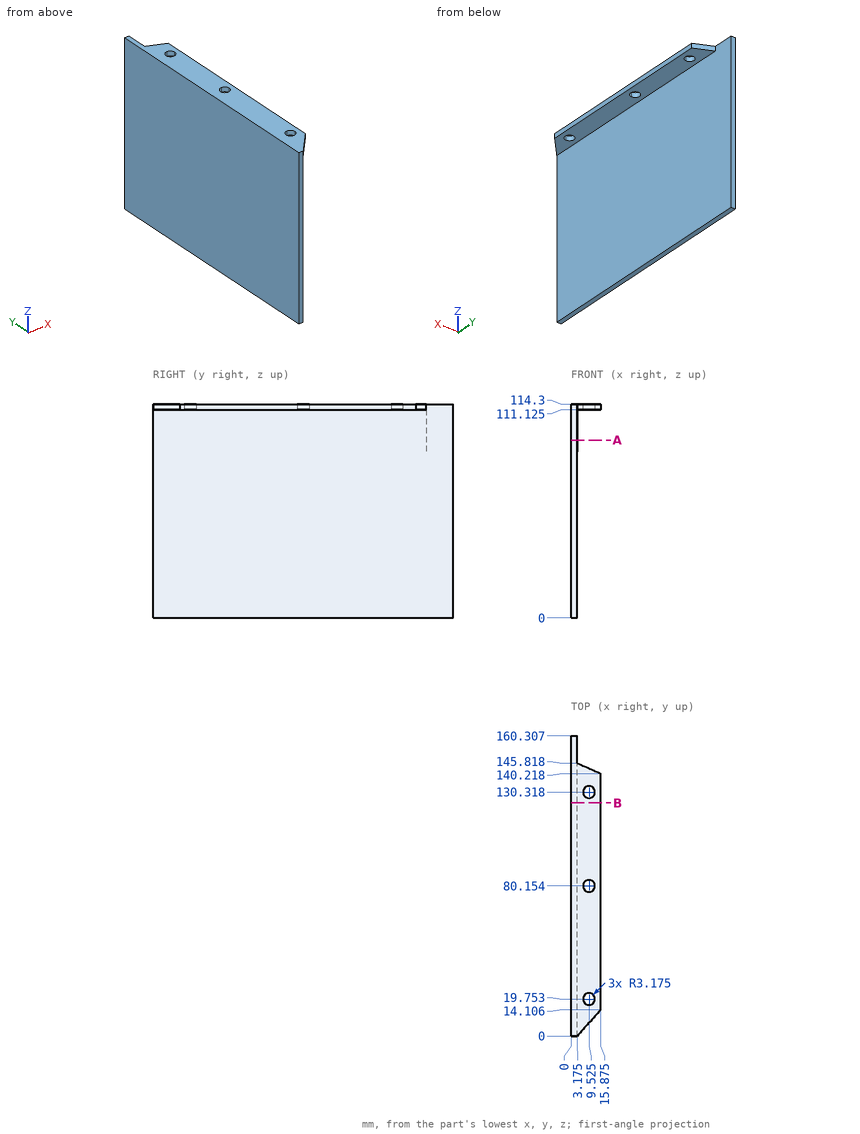
Can you work these out from the drawing? Everything is in mm from the part's minimum corner. Round coordinates to 2 decimals unless told otherwise and drop trailing zeros. Loops run counter-clockwise (first coordinate to the right, second up) from the corner with the lowest first, then second, coordinate; pieces in that order, holes last. Notation, with made-up numbers: (64, 84.25) - (92, 84.25) arc R13 ccw to (92, 99.25) - close; hole circle Ø10 at (22, -19). An arc over 180 degrees is marked (long way). Answer in a Markdown table with one row per item. Add a question column.
(1) I need wall thicknesses on line 1 along Z through (x, y) = (12.5, 121) (1 decimal); line 2 along X through (y, z) = (41.5, 58) (1 decimal). Which ranges of each line are inside material? Lowest first, please.
(2) If we section it at A-A (z = 95): Please give me the cut outline in (x, y) (1 decimal), plus the area to 3 significant figures.
(3) I'm going to push flat-ended pins straight in: pin 1 (10 mm diameter, centred on y = 23, z = 71.5, fed in from +X) (1 decimal); pin 2 (8 mm diameter, centred on x = 8, z = 39, fed in from -Y); pin 3 (6.5 mm diameter, centred on x = 8, y = 45.5, fed in from -Z) (1 decimal). Where does each tip first touch, or does it pass through?
(4) If we section it at B-B (y = 124.5): Please give me the cut outline in (x, z) (1 decimal), plus the area to 3 significant figures.
Model answer:
| question | item | result |
|---|---|---|
| 1 | line 1 | z = 111.1 to 114.3 |
| 1 | line 2 | x = 0 to 3.2 |
| 2 | outline | (0, 0) - (3.2, 0) - (3.2, 160.3) - (0, 160.3) - close |
| 2 | area | 509 mm² |
| 3 | pin 1 | stops at x = 3.2 |
| 3 | pin 2 | passes through |
| 3 | pin 3 | stops at z = 111.1 |
| 4 | outline | (0, 0) - (3.2, 0) - (3.2, 111.1) - (15.9, 111.1) - (15.9, 114.3) - (0, 114.3) - close |
| 4 | area | 403 mm² |
